from build123d import *
from OCP.BRepFilletAPI import BRepFilletAPI_MakeChamfer

# Parameters (mm, degrees)
T_LE_DE_BASE_PLI_E1_DEPTH       = 1.2
ESQUISSE12_R                    = 1.5
ESQUISSE12_R_2                  = 6
ENL_V_MAT_EXTRU_1_DEPTH         = 26.579729358
T_LE_START                      = -10.493561241
T_LE_PLI_E_SUR_AR_TE1_OUTLINE_W = 1.3366
T_LE_PLI_E_SUR_AR_TE1_OUTLINE_H = 1.2
T_LE_PLI_E_SUR_AR_TE1_DEPTH     = 0.6
T_LE_START_2                    = 9.540892015
T_LE_PLI_E_SUR_AR_TE1_2_DEPTH   = 0.6
T_LE_START_3                    = -9.893561241
T_LE_PLI_E_SUR_AR_TE1_3_DEPTH   = 19.434453256
T_LE_PLI_E_SUR_AR_TE1_4_DEPTH   = 2
T_LE_PLI_E_SUR_AR_TE1_5_DEPTH   = 19.434453256
T_LE_START_4                    = 16
T_LE_PLI_E_SUR_AR_TE1_6_DEPTH   = 1.2
T_LE_START_5                    = 2.2
T_LE_PLI_E_SUR_AR_TE2_DEPTH     = 27.8
T_LE_PLI_E_SUR_AR_TE2_2_DEPTH   = 0.6
T_LE_START_6                    = 2.8
T_LE_PLI_E_SUR_AR_TE2_3_DEPTH   = 27.2
CHANFREIN1_SIZE                 = 2
CHANFREIN1_SIZE2                = 5.740607303
CHANFREIN1_OF_SYM_TRIE1_SIZE    = 2
CHANFREIN1_OF_SYM_TRIE1_SIZE2   = 5.740607303
ENL_V_MAT_EXTRU_2_DEPTH         = 46.34668098
ENL_V_MAT_EXTRU_2_DEPTH_BACK    = 46.34668098
ENL_V_MAT_EXTRU_7_DEPTH         = 2


with BuildPart() as part:
    # Tôle de base pliée1: sheet metal written as solids
    # Esquisse1 → Tôle de base pliée1 (new body)
    with BuildSketch(Plane(origin=(0, 0, 0), x_dir=(1, 0, 0), z_dir=(0, 1, 0))):
        with BuildLine():
            Line((-5, 18.135119355), (-17.337811592, 4.837384541))
            ThreePointArc((-17.337811592, 4.837384541), (0, -18), (17.337811592, 4.837384541))
            Line((17.337811592, 4.837384541), (5, 18.135119355))
            Line((5, 18.135119355), (-5, 18.135119355))
        make_face()
    extrude(amount=-T_LE_DE_BASE_PLI_E1_DEPTH)

    # Esquisse12 → Enlèv. mat.-Extru.1 (cut, through all)
    with BuildSketch(Plane(origin=(0, 0, 0), x_dir=(1, 0, 0), z_dir=(0, 1, 0))):
        with Locations(Location((11, 0, 0), (0, 0, 270))):
            Circle(ESQUISSE12_R)
        with Locations(Location((0, 11, 0), (0, 0, 270))):
            Circle(ESQUISSE12_R)
        with Locations(Location((-11, 0, 0), (0, 0, 270))):
            Circle(ESQUISSE12_R)
        with Locations(Location((0, -11, 0), (0, 0, 270))):
            Circle(ESQUISSE12_R)
        with Locations(Location((0, 0, 0), (0, 0, 270))):
            Circle(ESQUISSE12_R_2)
    extrude(amount=-ENL_V_MAT_EXTRU_1_DEPTH, mode=Mode.SUBTRACT)

    # Tôle pliée sur arête1: read off the stored shape, not the designer's step
    # Tôle pliée sur arête1 outline → Tôle pliée sur arête1 (cut)
    with BuildSketch(Plane(origin=(0, 0, 0), x_dir=(0.7330706501266544, 0, -0.6801524990198037), z_dir=(0.6801524990198037, 0, 0.7330706501266546)).offset(T_LE_START)):
        with Locations((15.3317, -0.6)):
            Rectangle(T_LE_PLI_E_SUR_AR_TE1_OUTLINE_W, T_LE_PLI_E_SUR_AR_TE1_OUTLINE_H)
    t_le_pli_e_sur_ar_te1 = extrude(amount=T_LE_PLI_E_SUR_AR_TE1_DEPTH, mode=Mode.SUBTRACT)

    # T_le pli_e sur ar_te1 2 outline → T_le pli_e sur ar_te1 2 (cut)
    with BuildSketch(Plane(origin=(0, 0, 0), x_dir=(0.7330706501266544, 0, -0.6801524990198037), z_dir=(0.6801524990198037, 0, 0.7330706501266546)).offset(T_LE_START_2)):
        with BuildLine():
            Line((14.6634, 0), (14.6634, -1.2))
            Line((14.6634, -1.2), (15.2634, -1.2))
            ThreePointArc((15.2634, -1.2), (15.638821762, -1.163262642), (16, -1.054444388))
            Line((16, -1.054444388), (16, 0))
            Line((16, 0), (14.6634, 0))
        make_face()
    t_le_pli_e_sur_ar_te1_2 = extrude(amount=T_LE_PLI_E_SUR_AR_TE1_2_DEPTH, mode=Mode.SUBTRACT)

    # T_le pli_e sur ar_te1 3 outline → T_le pli_e sur ar_te1 3 (cut)
    with BuildSketch(Plane(origin=(0, 0, 0), x_dir=(0.7330706501266544, 0, -0.6801524990198037), z_dir=(0.6801524990198037, 0, 0.7330706501266546)).offset(T_LE_START_3)):
        with BuildLine():
            ThreePointArc((16, -1.054444388), (15.638821762, -1.163262642), (15.2634, -1.2))
            Line((15.2634, -1.2), (16, -1.2))
            Line((16, -1.2), (16, -1.054444388))
        make_face()
    t_le_pli_e_sur_ar_te1_3 = extrude(amount=T_LE_PLI_E_SUR_AR_TE1_3_DEPTH, mode=Mode.SUBTRACT)

    # T_le pli_e sur ar_te1 4 outline → T_le pli_e sur ar_te1 4 (add)
    with BuildSketch(Plane(origin=(0, 0, 0), x_dir=(0.7330706501266544, 0, -0.6801524990198037), z_dir=(0.6801524990198037, 0, 0.7330706501266546)).offset(T_LE_START_3)):
        with BuildLine():
            ThreePointArc((16, 0.7366), (15.784254855, 0.215745145), (15.2634, 0))
            Line((15.2634, 0), (16, 0))
            Line((16, 0), (16, -1.054444388))
            ThreePointArc((16, -1.054444388), (16.872269031, -0.341342484), (17.2, 0.7366))
            Line((17.2, 0.7366), (17.2, 30))
            Line((17.2, 30), (16, 30))
            Line((16, 30), (16, 0.7366))
        make_face()
    t_le_pli_e_sur_ar_te1_4 = extrude(amount=T_LE_PLI_E_SUR_AR_TE1_4_DEPTH)

    # T_le pli_e sur ar_te1 5 outline → T_le pli_e sur ar_te1 5 (add)
    with BuildSketch(Plane(origin=(0, 0, 0), x_dir=(0.7330706501266544, 0, -0.6801524990198037), z_dir=(0.6801524990198037, 0, 0.7330706501266546)).offset(T_LE_START_3)):
        with BuildLine():
            Line((14.6634, 0), (14.6634, -1.2))
            Line((14.6634, -1.2), (15.2634, -1.2))
            ThreePointArc((15.2634, -1.2), (16.632782992, -0.632782992), (17.2, 0.7366))
            Line((17.2, 0.7366), (16, 0.7366))
            ThreePointArc((16, 0.7366), (15.784254855, 0.215745145), (15.2634, 0))
            Line((15.2634, 0), (14.6634, 0))
        make_face()
    t_le_pli_e_sur_ar_te1_5 = extrude(amount=T_LE_PLI_E_SUR_AR_TE1_5_DEPTH)

    # T_le pli_e sur ar_te1 6 outline → T_le pli_e sur ar_te1 6 (add)
    with BuildSketch(Plane(origin=(0, 0, 0), x_dir=(0.6801524990198036, 0, 0.7330706501266546), z_dir=(0.7330706501266546, 0, -0.6801524990198037)).offset(T_LE_START_4)):
        Polygon((-7.893561241, -30), (9.508185371, -0.7366), (-7.893561241, -0.7366), align=None)
    t_le_pli_e_sur_ar_te1_6 = extrude(amount=T_LE_PLI_E_SUR_AR_TE1_6_DEPTH)

    # Tôle pliée sur arête2: read off the stored shape, not the designer's step
    # Tôle pliée sur arête2 outline → Tôle pliée sur arête2 (cut)
    with BuildSketch(Plane(origin=(0, 0, 0), x_dir=(1, 0, 0), z_dir=(0, 1, 0)).offset(T_LE_START_5)):
        with BuildLine():
            Line((5, 18.135119355), (5.516935379, 17.577964666))
            ThreePointArc((5.516935379, 17.577964666), (5.281888127, 17.88899285), (5.113898069, 18.240795467))
            Line((5.113898069, 18.240795467), (5, 18.135119355))
        make_face()
    t_le_pli_e_sur_ar_te2 = extrude(amount=T_LE_PLI_E_SUR_AR_TE2_DEPTH, mode=Mode.SUBTRACT)

    # T_le pli_e sur ar_te2 2 outline → T_le pli_e sur ar_te2 2 (cut)
    with BuildSketch(Plane(origin=(0, 0, 0), x_dir=(1, 0, 0), z_dir=(0, 1, 0)).offset(T_LE_START_5)):
        with BuildLine():
            Line((5.925026878, 17.138122276), (6.804711659, 17.954305274))
            Line((6.804711659, 17.954305274), (5.87968478, 18.951302354))
            Line((5.87968478, 18.951302354), (5.113898069, 18.240795467))
            ThreePointArc((5.113898069, 18.240795467), (5.281888127, 17.88899285), (5.516935379, 17.577964666))
            Line((5.516935379, 17.577964666), (5.925026878, 17.138122276))
        make_face()
    t_le_pli_e_sur_ar_te2_2 = extrude(amount=T_LE_PLI_E_SUR_AR_TE2_2_DEPTH, mode=Mode.SUBTRACT)

    # T_le pli_e sur ar_te2 3 outline → T_le pli_e sur ar_te2 3 (add)
    with BuildSketch(Plane(origin=(0, 0, 0), x_dir=(1, 0, 0), z_dir=(0, 1, 0)).offset(T_LE_START_6)):
        with BuildLine():
            Line((5.87968478, 18.951302354), (6.396620159, 18.394147664))
            ThreePointArc((6.396620159, 18.394147664), (6.250914682, 18.626047262), (6.2, 18.895147995))
            Line((6.2, 18.895147995), (6.2, 28.135119355))
            Line((6.2, 28.135119355), (5, 28.135119355))
            Line((5, 28.135119355), (5, 18.895147995))
            ThreePointArc((5, 18.895147995), (5.028686989, 18.563052376), (5.113898069, 18.240795467))
            Line((5.113898069, 18.240795467), (5.87968478, 18.951302354))
        make_face()
    t_le_pli_e_sur_ar_te2_3 = extrude(amount=T_LE_PLI_E_SUR_AR_TE2_3_DEPTH)

    # Chanfrein1: one chamfer whose edges measure the first distance from different faces: ONE call of the kernel's chamfer builder (chamfer() names one face for all edges)
    chanfrein1_edges_1 = [part.edges().sort_by_distance(p)[0] for p in [
        (5.6, 2.8, -28.135119355),
        (5.6, 30, -28.135119355),
    ]]
    chanfrein1_edges_2 = [part.edges().sort_by_distance(p)[0] for p in [
        (6.800147388, 30, -17.077069554),
    ]]
    chanfrein1_side_2 = [part.faces().sort_by_distance(p)[0] for p in [
        (5.687529449, 30, -22.422147631),
    ]]
    chanfrein1 = BRepFilletAPI_MakeChamfer(part.part.solid().wrapped)
    for e in chanfrein1_edges_1:
        chanfrein1.Add(CHANFREIN1_SIZE, e.wrapped)
    for e in chanfrein1_edges_2:
        chanfrein1.Add(CHANFREIN1_SIZE, CHANFREIN1_SIZE2, e.wrapped, chanfrein1_side_2[0].wrapped)  # the first distance lies on this face
    add(Compound.cast(chanfrein1.Shape()), mode=Mode.REPLACE)

    # Symétrie1: Tôle pliée sur arête1, T_le pli_e sur ar_te1 2, T_le pli_e sur ar_te1 3, T_le pli_e sur ar_te1 4, T_le pli_e sur ar_te1 5, T_le pli_e sur ar_te1 6, Tôle pliée sur arête2, T_le pli_e sur ar_te2 2, T_le pli_e sur ar_te2 3 across plane
    add(t_le_pli_e_sur_ar_te1.mirror(Plane(origin=(0, 0, 0), x_dir=(0, 0, 1), z_dir=(1, 0, 0))), mode=Mode.SUBTRACT)
    add(t_le_pli_e_sur_ar_te1_2.mirror(Plane(origin=(0, 0, 0), x_dir=(0, 0, 1), z_dir=(1, 0, 0))), mode=Mode.SUBTRACT)
    add(t_le_pli_e_sur_ar_te1_3.mirror(Plane(origin=(0, 0, 0), x_dir=(0, 0, 1), z_dir=(1, 0, 0))), mode=Mode.SUBTRACT)
    add(t_le_pli_e_sur_ar_te1_4.mirror(Plane(origin=(0, 0, 0), x_dir=(0, 0, 1), z_dir=(1, 0, 0))))
    add(t_le_pli_e_sur_ar_te1_5.mirror(Plane(origin=(0, 0, 0), x_dir=(0, 0, 1), z_dir=(1, 0, 0))))
    add(t_le_pli_e_sur_ar_te1_6.mirror(Plane(origin=(0, 0, 0), x_dir=(0, 0, 1), z_dir=(1, 0, 0))))
    add(t_le_pli_e_sur_ar_te2.mirror(Plane(origin=(0, 0, 0), x_dir=(0, 0, 1), z_dir=(1, 0, 0))), mode=Mode.SUBTRACT)
    add(t_le_pli_e_sur_ar_te2_2.mirror(Plane(origin=(0, 0, 0), x_dir=(0, 0, 1), z_dir=(1, 0, 0))), mode=Mode.SUBTRACT)
    add(t_le_pli_e_sur_ar_te2_3.mirror(Plane(origin=(0, 0, 0), x_dir=(0, 0, 1), z_dir=(1, 0, 0))))

    # Chanfrein1 of Symétrie1: one chamfer whose edges measure the first distance from different faces: ONE call of the kernel's chamfer builder (chamfer() names one face for all edges)
    chanfrein1_of_sym_trie1_edges_1 = [part.edges().sort_by_distance(p)[0] for p in [
        (-5.6, 2.8, -28.135119355),
        (-5.6, 30, -28.135119355),
    ]]
    chanfrein1_of_sym_trie1_edges_2 = [part.edges().sort_by_distance(p)[0] for p in [
        (-6.800147388, 30, -17.077069554),
    ]]
    chanfrein1_of_sym_trie1_side_2 = [part.faces().sort_by_distance(p)[0] for p in [
        (-5.687529449, 30, -22.422147631),
    ]]
    chanfrein1_of_sym_trie1 = BRepFilletAPI_MakeChamfer(part.part.solid().wrapped)
    for e in chanfrein1_of_sym_trie1_edges_1:
        chanfrein1_of_sym_trie1.Add(CHANFREIN1_OF_SYM_TRIE1_SIZE, e.wrapped)
    for e in chanfrein1_of_sym_trie1_edges_2:
        chanfrein1_of_sym_trie1.Add(CHANFREIN1_OF_SYM_TRIE1_SIZE, CHANFREIN1_OF_SYM_TRIE1_SIZE2, e.wrapped, chanfrein1_of_sym_trie1_side_2[0].wrapped)  # the first distance lies on this face
    add(Compound.cast(chanfrein1_of_sym_trie1.Shape()), mode=Mode.REPLACE)

    # Esquisse13 → Enlèv. mat.-Extru.2 (cut, two sides: drawn at the far end of the back side and taken through both)
    with BuildSketch(Plane(origin=(0, 0, 0), x_dir=(0, 0, -1), z_dir=(1, 0, 0)).offset(-ENL_V_MAT_EXTRU_2_DEPTH_BACK)):
        with BuildLine():
            Line((26.035119355, 23.4), (20.535119355, 23.4))
            ThreePointArc((20.535119355, 23.4), (18.935119355, 25), (20.535119355, 26.6))
            Line((20.535119355, 26.6), (26.035119355, 26.6))
            ThreePointArc((26.035119355, 26.6), (27.635119355, 25), (26.035119355, 23.4))
        make_face()
        with BuildLine():
            Line((26.035119355, 6.2), (20.535119355, 6.2))
            ThreePointArc((20.535119355, 6.2), (18.935119355, 7.8), (20.535119355, 9.4))
            Line((20.535119355, 9.4), (26.035119355, 9.4))
            ThreePointArc((26.035119355, 9.4), (27.635119355, 7.8), (26.035119355, 6.2))
        make_face()
    extrude(amount=ENL_V_MAT_EXTRU_2_DEPTH + ENL_V_MAT_EXTRU_2_DEPTH_BACK, mode=Mode.SUBTRACT)

    # Esquisse15 → Enlèv. mat.-Extru.7 (cut)
    with BuildSketch(Plane.XZ.offset(1.2)):
        Polygon((4.117844894, -17.316780768), (2.84424625, -16.135119355), (-2.84424625, -16.135119355), (-4.117844894, -17.316780768), (-4.117844894, -18.135119355), (4.117844894, -18.135119355), align=None)
    extrude(amount=-ENL_V_MAT_EXTRU_7_DEPTH, mode=Mode.SUBTRACT)


solid = part.part
Here's how the part is built. I have some questions about the finished solid (model axes, mm). A direction names the side the tool comes from. Give positions to 0.01 mm unless a question says otherwise; leave off trailing zeros. Order: outer loops, then holes, each group sorted by start corner. A loop starts at its lowest first (then second) coordinate and runs counter-clockwise, first axis right, second up. Notation, with made-up numbers: (20, 80) -> (40, 80) arc R23 cw to (40, 113) -> close; hole circle Ø11 at (-20, 35.5). An arc over 180 degrees is marked (long way). One line per item, written item: value. Start each with the question number.
1. Imagine slicing it at D-D, the plane z = 0. List the corners of the cut face in (x, y) for me, plus the area to 3 significant figures.
2. Imagine slicing it at A-A, the plane z = -25. List the corners of the cut face in (x, y) for me, plus the area to 3 significant figures.
3. Imagine slicing it at C-C, the plane y = 7.8. Count the separate pieces of the cut face and the enclosed holes in it, plus the area to 3 significant figures.
4. We'd pull the mould along X, two halves only. Please class faces 5 (the face through (6, 2.2, -18)), 6 (the face through (6.2, 16, -23)), 7 (the face through (-10.92, 11.62, -13.52)), 8 (the face through (6, 16, -28.135)): released by +X, released by -X, zero draft, split by the parting line, or undercut.
5. For faces 1 (the face through (-6, 9.4, -23)), 2 (the face through (-11.97, -0.65, -11.53)), 3 (the face through (18.155, -0.218, -3.83)), 4 (the face through (-11.36, 0.22, -10.97)), which set-ups out of +Z, -Z, +X, -X, +Y, -Y let a thin tool reach every point of the face, with its end or its side?
6. I need wall thicknesses on probe 1 along X at (y, z) = (-0.95, 0); probe 2 along X at (y, z) = (4, -21); probe 3 along Y at (x, z) = (-10.5, 9). Which ranges of each line are inside material? Lowest first, please. Write a range as from..to.
7. Imagine slicing it at B-B, the plane x = 0. List the corners of the cut face in (y, z) for me.
8. Will these pins go through, and if not, where does the flat tip stop? pin 1 Ø7.5 at (y, z) = (18.5, -25.5) entering from +X; pin 2 Ø10 at (y, z) = (18.5, -24.5) entering from -X; pin 3 Ø15.5 at (x, z) = (0, 0) entering from +Y.
Values follow:
1. outline: (-18, -1.2) -> (-12.5, -1.2) -> (-12.5, 0) -> (-18, 0) -> close; (-9.5, -1.2) -> (-6, -1.2) -> (-6, 0) -> (-9.5, 0) -> close; (6, -1.2) -> (9.5, -1.2) -> (9.5, 0) -> (6, 0) -> close; (12.5, -1.2) -> (18, -1.2) -> (18, 0) -> (12.5, 0) -> close
1. area: 21.6 mm2
2. outline: (-6.2, 2.8) -> (-5, 2.8) -> (-5, 6.2) -> (-6.2, 6.2) -> close; (-6.2, 9.4) -> (-5, 9.4) -> (-5, 23.4) -> (-6.2, 23.4) -> close; (-6.2, 26.6) -> (-5, 26.6) -> (-5, 30) -> (-6.2, 30) -> close; (5, 2.8) -> (6.2, 2.8) -> (6.2, 6.2) -> (5, 6.2) -> close; (5, 9.4) -> (6.2, 9.4) -> (6.2, 23.4) -> (5, 23.4) -> close; (5, 26.6) -> (6.2, 26.6) -> (6.2, 30) -> (5, 30) -> close
2. area: 49.9 mm2
3. separate pieces: 4
3. enclosed holes: 0
3. area: 38.4 mm2
4. face 5: undercut
4. face 6: released by +X
4. face 7: released by -X
4. face 8: zero draft
5. face 1: +X, -X
5. face 2: -Z, -X, -Y
5. face 3: +X, +Y, -Y
5. face 4: +Z, +Y
6. probe 1: x = -18..-12.5, -9.5..-6, 6..9.5, 12.5..18
6. probe 2: x = -6.2..-5, 5..6.2
6. probe 3: y = -1.2..0
7. outline: (-1.2, -16.14) -> (0, -16.14) -> (0, -12.5) -> (-1.2, -12.5) -> close; (-1.2, -9.5) -> (0, -9.5) -> (0, -6) -> (-1.2, -6) -> close; (-1.2, 6) -> (0, 6) -> (0, 9.5) -> (-1.2, 9.5) -> close; (-1.2, 12.5) -> (0, 12.5) -> (0, 18) -> (-1.2, 18) -> close
8. pin 1: stops at x = 6.2
8. pin 2: stops at x = -6.2
8. pin 3: stops at y = 0
